```python
from build123d import *

# Parameters (mm, degrees)
SKETCH1_W             = 20
SKETCH1_H             = 34
SKETCH1_R             = 2.75
BOSS_EXTRUDE1_DEPTH   = 2
SKETCH2_W             = 10
SKETCH2_H             = 34
BOSS_EXTRUDE2_DEPTH   = 2
BOSS_EXTRUDE2_2_DEPTH = 2
SKETCH3_W             = 10
SKETCH3_H             = 34
BOSS_EXTRUDE3_DEPTH   = 7
SKETCH4_W             = 20.4
SKETCH4_H             = 2
BOSS_EXTRUDE4_DEPTH   = 34
CUT_EXTRUDE2_DEPTH    = 41.162669234
SKETCH6_R             = 2.75
CUT_EXTRUDE3_DEPTH    = 66.582314689


with BuildPart() as part:
    # Sketch1 → Boss-Extrude1 (new body)
    with BuildSketch(Plane.XY):
        with Locations((0, 45)):
            Rectangle(SKETCH1_W, SKETCH1_H)
        with Locations((0, 32)):
            Circle(SKETCH1_R, mode=Mode.SUBTRACT)
        with Locations((0, 52)):
            Circle(SKETCH1_R, mode=Mode.SUBTRACT)
    extrude(amount=BOSS_EXTRUDE1_DEPTH)



with BuildPart() as body_2:
    # Sketch2 → Boss-Extrude2 (new body)
    with BuildSketch(Plane(origin=(0, 0, 0), x_dir=(-1, 0, 0), z_dir=(0, 0, -1))):
        with Locations((15.2, 45)):
            Rectangle(SKETCH2_W, SKETCH2_H)
    extrude(amount=-BOSS_EXTRUDE2_DEPTH)



with BuildPart() as body_3:
    # Sketch2 → Boss-Extrude2 2 (new body)
    with BuildSketch(Plane(origin=(0, 0, 0), x_dir=(-1, 0, 0), z_dir=(0, 0, -1))):
        with Locations((-15.2, 45)):
            Rectangle(SKETCH2_W, SKETCH2_H)
    extrude(amount=-BOSS_EXTRUDE2_2_DEPTH)


with BuildPart() as body_2_1:
    add(body_2.part)

    add(body_3.part)  # Boss-Extrude3 merges body 3
    # Sketch3 → Boss-Extrude3 (add)
    with BuildSketch(Plane(origin=(0, 0, 0), x_dir=(-1, 0, 0), z_dir=(0, 0, -1))):
        with Locations((-15.2, 45)):
            Rectangle(SKETCH3_W, SKETCH3_H)
        with Locations((15.2, 45)):
            Rectangle(SKETCH3_W, SKETCH3_H)
    extrude(amount=BOSS_EXTRUDE3_DEPTH)


with BuildPart() as part_1:
    add(part.part)

    add(body_2_1.part)  # Boss-Extrude4 merges body 2
    # Sketch4 → Boss-Extrude4 (add)
    with BuildSketch(Plane(origin=(0, 62, 0), x_dir=(1, 0, 0), z_dir=(0, 1, 0))):
        with Locations((0, -1)):
            Rectangle(SKETCH4_W, SKETCH4_H)
    extrude(amount=-BOSS_EXTRUDE4_DEPTH)

    # Sketch5 → Cut-Extrude2 (cut, through all)
    with BuildSketch(Plane(origin=(0, 62, 0), x_dir=(1, 0, 0), z_dir=(0, 1, 0))):
        Polygon((12.2, 0), (12.2, -2), (20.2, -2), (20.2, 5), (12.2, 5), align=None)
        Polygon((-12.2, -2), (-12.2, 0), (-12.2, 5), (-20.2, 5), (-20.2, -2), align=None)
    extrude(amount=-CUT_EXTRUDE2_DEPTH, mode=Mode.SUBTRACT)

    # Sketch6 → Cut-Extrude3 (cut, through all)
    with BuildSketch(Plane(origin=(0, 0, 0), x_dir=(-1, 0, 0), z_dir=(0, 0, -1))):
        with Locations((0, 52)):
            Circle(SKETCH6_R)
        with Locations((0, 32)):
            Circle(SKETCH6_R)
    extrude(amount=-CUT_EXTRUDE3_DEPTH, mode=Mode.SUBTRACT)


solid = part_1.part
```
The model under review builds one solid part; all positions refer to its coordinate system, in mm. A direction names the side the tool comes from. Round coordinates to 2 decimals unless told otherwise and drop trailing zeros. Order: outer loops, then holes, each group sorted by start corner. A loop starts at its lowest first (then second) coordinate and runs counter-clockwise, first axis right, second up. Notation, with made-up numbers: (-32.5, 73.5) -> (4.5, 73.5) arc R11 cw to (4.5, 88.5) -> close; hole circle Ø9 at (53.25, 16.5). An arc over 180 degrees is marked (long way). One line per item, written item: value. Start each with the question number.
Q1. Take a section at C-C (x = 0). Write out the cut boundary in (y, z), and give its area (3 significant figures).
Q2. Take a section at B-B (z = -1). Write out the cut boundary in (x, y).
Q3. Take a section at D-D (y = 37.5). Write out the cut boundary in (x, z).
Q4. Mouldability with a two-part tool opening along X and no side actions: class faces 1 (the face through (-12.2, 45, -1)), 2 (the face through (-16, 45, -5)), 3 (the face through (0.358, 54.727, 0.986)), 4 (the face through (-10.2, 45, -3)) as released by +X, released by -X, zero draft, split by the parting line, or undercut.
Q5. Wall thickness on line 1 (Y direction, x = 0, z = 1.4); line 2 (X direction, y = 59.5, z = -0.5); line 3 (Z direction, x = -9.5, y = 31.5): over which ranges is each line inside the solid? List them lowest first.
Q6. Clearance check with flat-ended pins moving along their axes: pin 1 Ø4 at (x, z) = (7, -5) entering from +Y; pin 2 Ø2 at (y, z) = (47, -3.5) entering from +X; pin 3 Ø1.5 at (y, z) = (47, -2) entering from -X; pin 4 Ø6.5 at (x, y) = (16.5, 49.5) entering from +Z. State where each tip first meets the part, or that it passes through.
Q7. Take a section at A-A (y = 32). Write out the cut boundary in (x, z).
Q8. Machinability: for faces 5 (the face through (16, 45, -5)), 6 (the face through (0, 62, 1)), 7 (the face through (10.2, 45, -3)), which of the approach directions +Z, -Z, +X, -X, +Y, -Y give a long, thin tool a straight path to every point of the face, cutting with its end or side? Answer none if there is none.
Reported:
1. outline: (28, 0) -> (29.25, 0) -> (29.25, 2) -> (28, 2) -> close; (34.75, 0) -> (49.25, 0) -> (49.25, 2) -> (34.75, 2) -> close; (54.75, 0) -> (62, 0) -> (62, 2) -> (54.75, 2) -> close
1. area: 46.0 mm2
2. outline: (-12.2, 28) -> (-10.2, 28) -> (-10.2, 62) -> (-12.2, 62) -> close; (10.2, 28) -> (12.2, 28) -> (12.2, 62) -> (10.2, 62) -> close
3. outline: (-20.2, -7) -> (-10.2, -7) -> (-10.2, 0) -> (10.2, 0) -> (10.2, -7) -> (20.2, -7) -> (20.2, -5) -> (12.2, -5) -> (12.2, 2) -> (-12.2, 2) -> (-12.2, -5) -> (-20.2, -5) -> close
4. face 1: released by -X
4. face 2: zero draft
4. face 3: undercut
4. face 4: undercut
5. line 1: y = 28 to 29.25, 34.75 to 49.25, 54.75 to 62
5. line 2: x = -12.2 to -10.2, 10.2 to 12.2
5. line 3: z = 0 to 2
6. pin 1: passes through
6. pin 2: stops at x = 12.2
6. pin 3: stops at x = -12.2
6. pin 4: stops at z = -5
7. outline: (-20.2, -7) -> (-10.2, -7) -> (-10.2, 0) -> (-2.75, 0) -> (-2.75, 2) -> (-12.2, 2) -> (-12.2, -5) -> (-20.2, -5) -> close; (2.75, 0) -> (10.2, 0) -> (10.2, -7) -> (20.2, -7) -> (20.2, -5) -> (12.2, -5) -> (12.2, 2) -> (2.75, 2) -> close
8. face 5: +Z, +X, +Y, -Y
8. face 6: +Z, -Z, +X, -X, +Y
8. face 7: -Z, +Y, -Y
